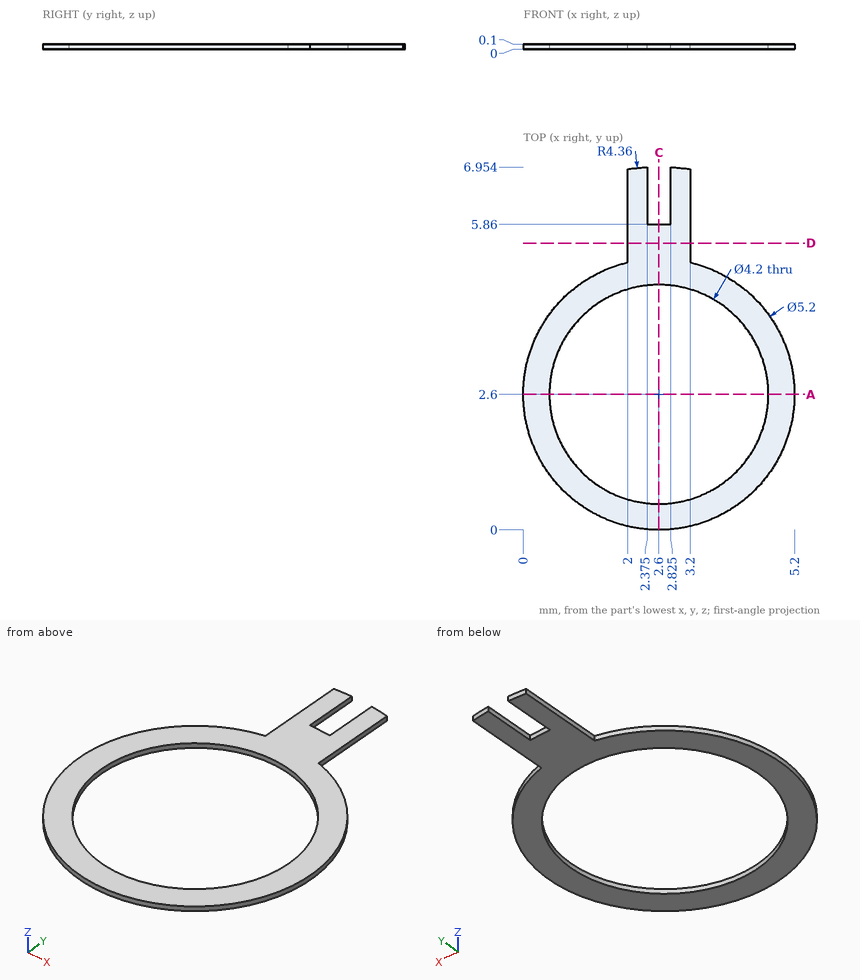
The figure shows three views and two pictorial views of one solid part (mm, origin at its lowest corner). Answer the questions. Round coordinates to 2 decimals unless told otherwise and drop trailing zeros. Write each loop counter-clockwise with the first axis right and the second up, starting at its lowest first coordinate (ties: lowest second). Pieces come first, ordered by that corner, then holes. Notation, with made-up numbers: (-7, -5.75) - (13, -5.75) arc R36 ccw to (13, 28.25) - close; hole circle Ø6 at (-34.75, 85). An arc over 180 degrees is marked (long way). Use one line per item in the form item = value. Start each with the question number.
Item 1: A cutting plane is placed at A-A (y = 2.6). Write down the section's boundary in (x, z).
Item 2: Find the intervals of material crossed by line 1 (X direction, y = 3.25, z = 0.05); line 2 (Y direction, x = 0.85, z = 0.05); line 3 (Y direction, x = 4.15, z = 0.05), in increasing order. Write a range as [from, to].
Item 3: A cutting plane is placed at D-D (y = 5.5). Write down the section's boundary in (x, z).
Item 4: A cutting plane is placed at C-C (x = 2.6). Write down the section's boundary in (y, z).
The answers:
q1.outline = (0, 0) - (0.5, 0) - (0.5, 0.1) - (0, 0.1) - close; (4.7, 0) - (5.2, 0) - (5.2, 0.1) - (4.7, 0.1) - close
q2.line_1 = [0.08, 0.6], [4.6, 5.12]
q2.line_2 = [0.68, 1.44], [3.76, 4.52]
q2.line_3 = [0.51, 1.18], [4.02, 4.69]
q3.outline = (2, 0) - (3.2, 0) - (3.2, 0.1) - (2, 0.1) - close
q4.outline = (0, 0) - (0.5, 0) - (0.5, 0.1) - (0, 0.1) - close; (4.7, 0) - (5.86, 0) - (5.86, 0.1) - (4.7, 0.1) - close
